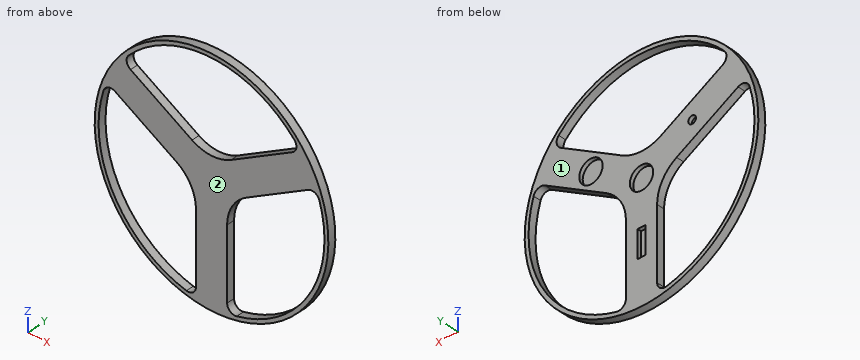
```python
from build123d import *

# Parameters (mm, degrees)
SKETCH1_R           = 30
BOSS_EXTRUDE1_DEPTH = 2
FILLET1_R           = 10
FILLET2_R           = 2
SKETCH2_R           = 3
CUT_EXTRUDE1_DEPTH  = 1
SKETCH3_R           = 1
SKETCH3_R_2         = 3
SKETCH3_W           = 2
SKETCH3_H           = 7
CUT_EXTRUDE2_DEPTH  = 1


with BuildPart() as part:
    # Sketch1 → Boss-Extrude1 (new body)
    with BuildSketch(Plane(origin=(0, 0, 0), x_dir=(1, 0, 0), z_dir=(0, 1, 0))):
        with Locations(Location((0, 0, 0), (0, 0, 270))):
            Circle(SKETCH1_R)
        with BuildLine():
            Line((-22.874685928, -17.825508231), (0, -4.618802154))
            Line((0, -4.618802154), (22.874685928, -17.825508231))
            ThreePointArc((22.874685928, -17.825508231), (0, -29), (-22.874685928, -17.825508231))
        make_face(mode=Mode.SUBTRACT)
        with BuildLine():
            Line((26.874685928, -10.897305001), (4, 2.309401077))
            Line((4, 2.309401077), (4, 28.722813233))
            ThreePointArc((4, 28.722813233), (25.11473671, 14.5), (26.874685928, -10.897305001))
        make_face(mode=Mode.SUBTRACT)
        with BuildLine():
            Line((-4, 28.722813233), (-4, 2.309401077))
            Line((-4, 2.309401077), (-26.874685928, -10.897305001))
            ThreePointArc((-26.874685928, -10.897305001), (-25.11473671, 14.5), (-4, 28.722813233))
        make_face(mode=Mode.SUBTRACT)
    extrude(amount=BOSS_EXTRUDE1_DEPTH)

    # Fillet1
    fillet1_edges = [part.edges().sort_by_distance(p)[0] for p in [
        (0, 1, 4.618802154),
        (-4, 1, -2.309401077),
        (4, 1, -2.309401077),
    ]]
    fillet(fillet1_edges, radius=FILLET1_R)

    # Fillet2
    fillet2_edges = [part.edges().sort_by_distance(p)[0] for p in [
        (-22.874685928, 1, 17.825508231),
        (22.874685928, 1, 17.825508231),
        (-4, 1, -28.722813233),
        (-26.874685928, 1, 10.897305001),
        (26.874685928, 1, 10.897305001),
        (4, 1, -28.722813233),
    ]]
    fillet(fillet2_edges, radius=FILLET2_R)

    # Sketch2 → Cut-Extrude1 (cut)
    with BuildSketch(Plane(origin=(0, 2, 0), x_dir=(1, 0, 0), z_dir=(0, 1, 0))):
        with Locations(Location((0, 0, 0), (0, 0, 270))):
            Circle(SKETCH2_R)
    extrude(amount=-CUT_EXTRUDE1_DEPTH, mode=Mode.SUBTRACT)

    # Sketch3 → Cut-Extrude2 (cut)
    with BuildSketch(Plane(origin=(0, 2, 0), x_dir=(1, 0, 0), z_dir=(0, 1, 0))):
        with Locations(Location((-12.990200407, -7.500312817, 0), (0, 0, 270))):
            Circle(SKETCH3_R)
        with Locations(Location((12.990019825, -7.499374327, 0), (0, 0, 270))):
            Circle(SKETCH3_R_2)
        with Locations((-0.000361232, 15.000625673)):
            Rectangle(SKETCH3_W, SKETCH3_H)
    extrude(amount=-CUT_EXTRUDE2_DEPTH, mode=Mode.SUBTRACT)


solid = part.part
```
Here's how the part is built. I have some questions about the finished solid (model axes, mm). Face numbers are marked on the shaded views. Give positions to 0.01 mm unless a question says otherwise; leave off trailing zeros. Loops run counter-clockwise (first coordinate to the right, second up) from the corner with the lowest first, then second, coordinate; pieces in that order, holes last. Notation, with made-up numbers: M 87.5,-18.5 L 107.5,-18.5 A15 cw 107.5,-6.5 Z; hole C -19.75,86 d4. An arc over 180 degrees is marked long. Return JSON: item names as keys, results as strings.
Item 1: Imagine slicing it at A-A on x = 0. List the corners of the cut face in (y, z) for me.
A:
{"outline": "M 0,-30 L 2,-30 L 2,-18.5 L 1,-18.5 L 1,-11.5 L 2,-11.5 L 2,-3 L 1,-3 L 1,3 L 2,3 L 2,6.17 L 0,6.17 Z; M 0,29 L 2,29 L 2,30 L 0,30 Z"}
Item 2: Please list where these lines run through material, in increasing order: line 1 (X direction, y = 1.6, z = 8); line 2 (Z direction, x = 19.5, y = 1.2); line 3 (X direction, y = 0.45, z = 2).
A:
{"line 1": "x = -28.91 to -27.87, -21.86 to -13.86, -12.12 to -5.86, 5.86 to 10.03, 15.95 to 21.86, 27.87 to 28.91", "line 2": "z = -22.8 to -21.47, 6.64 to 15.88, 21.47 to 22.8", "line 3": "x = -29.93 to -28.93, -11.46 to 11.46, 28.93 to 29.93"}
Item 3: Imagine slicing it at C-C on x = 19. List the corners of the cut face in (y, z) for me, then the cut area to 3 significant figures.
A:
{"outline": "M 0,-23.22 L 2,-23.22 L 2,-21.91 L 0,-21.91 Z; M 0,6.35 L 2,6.35 L 2,15.59 L 0,15.59 Z; M 0,21.91 L 2,21.91 L 2,23.22 L 0,23.22 Z", "area": "23.7 mm^2"}
Item 4: Imagine slicing it at D-D on y = 1.3. List the corners of the cut face in (x, z) for me.
A:
{"outline": "C 0,0 d60; hole M -27.71,8.56 A29 ccw -6.44,-28.27 A2 ccw -4,-26.32 L -4,-8.08 A10 ccw -9,0.58 L -24.8,9.7 A2 ccw Z; hole M -21.26,19.72 A2 ccw -20.8,16.63 L -5,7.51 A10 ccw 5,7.51 L 20.8,16.63 A2 ccw 21.26,19.72 A29 ccw Z; hole C -12.99,7.5 d2; hole C 0,0 d6; hole M -1,-18.5 L 1,-18.5 L 1,-11.5 L -1,-11.5 Z; hole M 4,-26.32 A2 ccw 6.44,-28.27 A29 ccw 27.71,8.56 A2 ccw 24.8,9.7 L 9,0.58 A10 ccw 4,-8.08 Z; hole C 12.99,7.5 d6"}
Item 5: Imagine slicing it at B-B on z = -5. List the corners of the cut face in (x, y) for me, then the cut area to 3 significant figures.
A:
{"outline": "M -29.58,0 L -28.57,0 L -28.57,2 L -29.58,2 Z; M -4.49,0 L 4.49,0 L 4.49,2 L -4.49,2 Z; M 28.57,0 L 29.58,0 L 29.58,2 L 28.57,2 Z", "area": "22.0 mm^2"}
Item 6: Thinking about a two-plate mould opening in Y: for the marked faces 1 and 2, which applies, released by +Y, released by -Y, zero draft, split by the parting line, or undercut?
A:
{"face 1": "released by +Y", "face 2": "released by -Y"}
Item 7: I'm going to push flat-ended pins straight in: pin 1 Ø1 at (y, z) = (1.5, -21) entering from -X; pin 2 Ø1 at (x, y) = (-5, 1.5) entering from +Z; pin 3 Ø1.1 at (y, z) = (1.5, -14.5) entering from +X. Where does each tip first touch, or does it pass through?
A:
{"pin 1": "stops at x = -21.9", "pin 2": "stops at z = 29.66", "pin 3": "stops at x = 26.56"}
